Check sheet for the drawn part. Datum: minimum x, y, z corner. Units: mm. Coordinates: 2 decimals unless noted, no trailing zeros. Order: outer loops, then holes, each group sorted by start corner. A loop starts at its lowest first (then second) coordinate and runs counter-clockwise, first axis right, second up. Notation, with made-up numbers: (60.5, -8.5) - (96.5, -8.5) arc R19 ccw to (96.5, 28.5) - close; hole circle Ø4 at (-12, -20). An arc over 180 degrees is marked (long way). Return JSON: item names as keys, results as strings. Group by question number.
Item 1: Scan lines: probe 1 along X at (y, z) = (69, 1.7); probe 2 along Y at (x, z) = (24.5, 0.4) (3 decimals); probe 3 along X at (y, z) = (53, 1.05). Record each from-to range of solid material in increasing order.
Item 2: Section check D-D on y = 70. Enter the section's corners in (x, z).
Item 3: Section check A-A on y = 48.5. Enter the section's corners in (x, z), then the cut area to 3 significant figures.
Item 4: Section check C-C on x = 62. Enter the section's corners in (y, z), then the cut area to 3 significant figures.
Item 5: Gauge pin test, flat ends, axial feed: pin 1 (0.9 mm diameter, centred on x = 37.5, z = 1, fed in from +Y); pin 2 (1.5 mm diameter, centred on y = 69.5, z = 1.5, fed in from +X). Record the tip position at first contact, or that the pin passes through.
Item 6: Section check B-B on z = 1.3. Enter the section's corners in (x, y) (3 decimals), then the cut area to 3 significant figures.
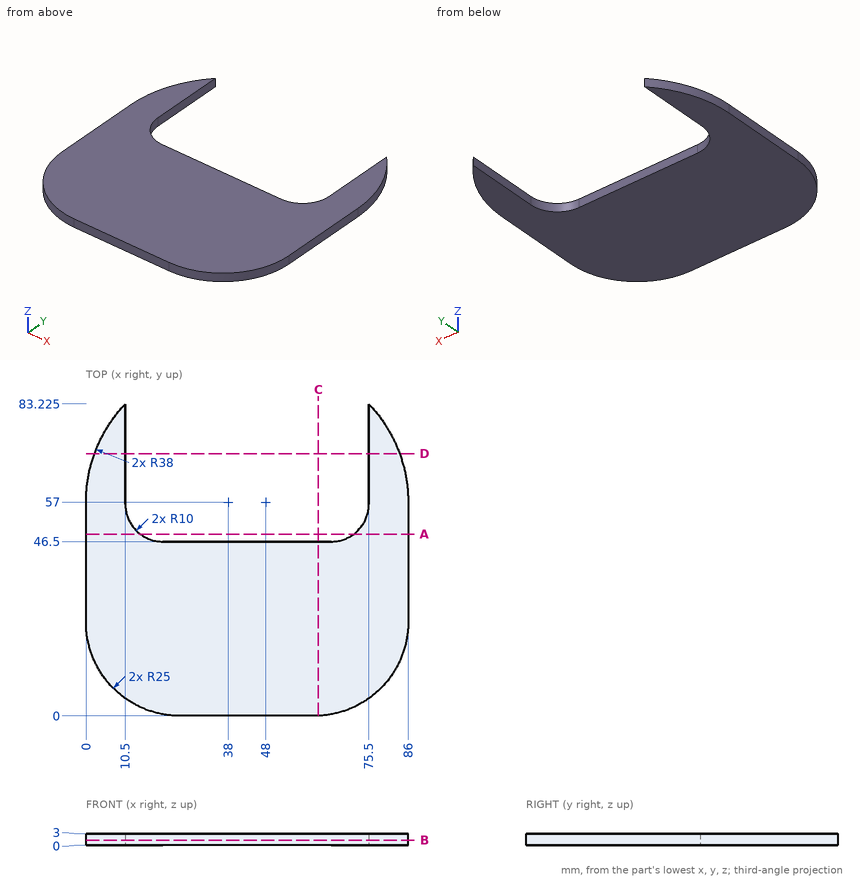
Computed:
{
 "1": {"probe 1": "x = 1.94 to 10.5, 75.5 to 84.06", "probe 2": "y = 0.005 to 46.5", "probe 3": "x = 0 to 11.13, 74.87 to 86"},
 "2": {"outline": "(2.29, 0) - (10.5, 0) - (10.5, 3) - (2.29, 3) - close; (75.5, 0) - (83.71, 0) - (83.71, 3) - (75.5, 3) - close"},
 "3": {"outline": "(0, 0) - (14.5, 0) - (14.5, 3) - (0, 3) - close; (71.5, 0) - (86, 0) - (86, 3) - (71.5, 3) - close", "area": "87.0 mm²"},
 "4": {"outline": "(0.02, 0) - (46.5, 0) - (46.5, 3) - (0.02, 3) - close", "area": "139 mm²"},
 "5": {"pin 1": "stops at y = 46.5", "pin 2": "stops at x = 84.14"},
 "6": {"outline": "(0, 25) arc R25 ccw to (25, 0) - (61, 0) arc R25 ccw to (86, 25) - (86, 57) arc R38 ccw to (75.5, 83.225) - (75.5, 56.5) arc R10 cw to (65.5, 46.5) - (20.5, 46.5) arc R10 cw to (10.5, 56.5) - (10.5, 83.225) arc R38 ccw to (0, 57) - close", "area": "4,370 mm²"}
}
